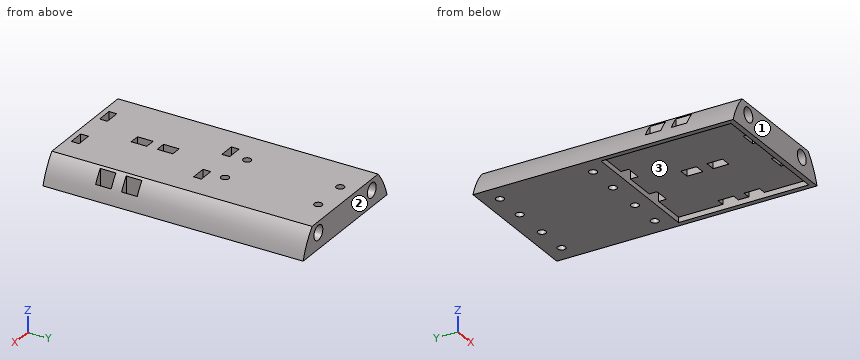
from build123d import *

# Parameters (mm, degrees)
BOSS_EXTRUDE1_DEPTH       = 127
SKETCH10_W                = 62.671930198
SKETCH10_H                = 63.5
CUT_EXTRUDE1_DEPTH        = 2.54
F_1_4_CLEARANCE_HOLE1_D   = 7.14248
F_8_CLEARANCE_HOLE1_D     = 3.8608
SKETCH19_W                = 5.08
SKETCH19_H                = 7.62
SKETCH19_W_2              = 3.81
SKETCH19_W_3              = 7.62
SKETCH19_H_2              = 3.81
CUT_EXTRUDE3_DEPTH        = 14.188436542
F_8_CLEARANCE_HOLE2_D     = 3.8608
F_8_CLEARANCE_HOLE2_DEPTH = 3.81


with BuildPart() as part:
    # Sketch1 → Boss-Extrude1 (new body)
    with BuildSketch(Plane(origin=(0, 0, 0), x_dir=(1, 0, 0), z_dir=(0, 1, 0))):
        with BuildLine():
            Line((-33.875965099, -9.946488053), (33.875965099, -9.946488053))
            ThreePointArc((33.875965099, -9.946488053), (30.982853114, -16.928569016), (26.67, -23.134924595))
            Line((26.67, -23.134924595), (-26.67, -23.134924595))
            ThreePointArc((-26.67, -23.134924595), (-30.982853114, -16.928569016), (-33.875965099, -9.946488053))
        make_face()
    extrude(amount=BOSS_EXTRUDE1_DEPTH)

    # Sketch10 → Cut-Extrude1 (cut)
    with BuildSketch(Plane(origin=(0, 0, 9.946488053), x_dir=(-1, 0, 0), z_dir=(0, 0, -1))):
        with Locations((0, 34.29)):
            Rectangle(SKETCH10_W, SKETCH10_H)
    extrude(amount=-CUT_EXTRUDE1_DEPTH, mode=Mode.SUBTRACT)

    # 1/4 Clearance Hole1 (through all)
    with Locations(Plane(origin=(0, 127, 0), x_dir=(1, 0, 0), z_dir=(0, 1, 0))):
        with Locations((-21.59, -17.810706324), (21.59, -17.810706324)):
            Hole(F_1_4_CLEARANCE_HOLE1_D / 2)

    # #8 Clearance Hole1 (through all)
    with Locations(Plane(origin=(0, 0, 9.946488053), x_dir=(-1, 0, 0), z_dir=(0, 0, -1))):
        with Locations((-8.93698255, 119.253), (-8.93698255, 73.787), (8.93698255, 73.787), (8.93698255, 119.253)):
            Hole(F_8_CLEARANCE_HOLE1_D / 2)

    # Sketch19 → Cut-Extrude3 (cut, through all)
    with BuildSketch(Plane(origin=(0, 0, 9.946488053), x_dir=(-1, 0, 0), z_dir=(0, 0, -1))):
        with Locations((0, 40.64)):
            Rectangle(SKETCH19_W, SKETCH19_H)
        with Locations((0, 27.94)):
            Rectangle(SKETCH19_W, SKETCH19_H)
        with Locations((29.430965099, 40.64)):
            Rectangle(SKETCH19_W_2, SKETCH19_H)
        with Locations((-11.43, 64.135)):
            Rectangle(SKETCH19_W_3, SKETCH19_H_2)
        with Locations((11.43, 64.135)):
            Rectangle(SKETCH19_W_3, SKETCH19_H_2)
        with Locations((-11.43, 4.445)):
            Rectangle(SKETCH19_W_3, SKETCH19_H_2)
        with Locations((11.43, 4.445)):
            Rectangle(SKETCH19_W_3, SKETCH19_H_2)
        with Locations((-29.430965099, 40.64)):
            Rectangle(SKETCH19_W_2, SKETCH19_H)
        with Locations((29.430965099, 27.94)):
            Rectangle(SKETCH19_W_2, SKETCH19_H)
        with Locations((-29.430965099, 27.94)):
            Rectangle(SKETCH19_W_2, SKETCH19_H)
    extrude(amount=-CUT_EXTRUDE3_DEPTH, mode=Mode.SUBTRACT)

    # #8 Clearance Hole2
    with Locations(Plane(origin=(0, 0, 9.946488053), x_dir=(-1, 0, 0), z_dir=(0, 0, -1))):
        with Locations((-24.93898255, 119.253), (-24.93898255, 73.787), (24.93898255, 73.787), (24.93898255, 119.253)):
            Hole(F_8_CLEARANCE_HOLE2_D / 2, depth=F_8_CLEARANCE_HOLE2_DEPTH)


solid = part.part
Geometry: final body of the model. Coordinates: model frame, mm. Face numbers are marked on the shaded views. Give positions to 0.01 mm unless a question says otherwise; leave off trailing zeros. Write each loop counter-clockwise with the first axis right and the second up, starting at its lowest first coordinate (ties: lowest second). Pieces come first, ordered by that corner, then holes. Notation, with made-up numbers: M 68.25,6 L 72.25,6 A24 ccw 72.25,16 Z; hole C -28.75,68 d4. An arc over 180 degrees is marked long. Answer in a Markdown table with one row per item. Add a question column.
(1) First-contact query: pin 1 (6 mm diameter, centred on y = 39.5, z = 20, fed in from +X); pin 2 (2.5 mm diameter, centred on x = 24.94, y = 73.79, fed in from -Z); pin 3 (7 mm diameter, centred on y = 35.5, z = 11.5, fed in from +X). Flat tips, straight axial feed; report the tip coordinate or a pass-through.
(2) Mould query, pull axis Y, two halves, no side actions, for the marked faces 1, 2 and 3. Classes: +Y half, -Y half, draft (parallel to the pull), parting line (faces both ways), or undercut.
(3) Section B-B on y = 41.5. Return loops of the section in (x, z), and give its area (3 significant figures).
(4) Ray query, line 1 (Y direction, x = -0.5, z = 16.75); line 2 (X direction, y = 26.5, z = 17.5); line 3 (Y direction, x = -12, z = 22). Return the intervals inside material, ascending.
(5) Section C-C on x = 0. Return loops of the section in (y, z).
(6) Section D-D on y = 55. Return loops of the section in (x, z).
(7) Section A-A on x = 21.59. Return loops of the section in (y, z), and give its area (3 significant figures).
Result set:
| question | item | result |
|---|---|---|
| 1 | pin 1 | stops at x = 29.99 |
| 1 | pin 2 | stops at z = 13.76 |
| 1 | pin 3 | stops at x = 33.88 |
| 2 | face 1 | -Y half |
| 2 | face 2 | +Y half |
| 2 | face 3 | undercut |
| 3 | outline | M -33.88,9.95 L -31.34,9.95 L -31.34,16.27 A35.31 ccw Z; M -27.53,12.49 L -2.54,12.49 L -2.54,23.13 L -26.67,23.13 A35.31 ccw -27.53,22.11 Z; M 2.54,12.49 L 27.53,12.49 L 27.53,22.11 A35.31 ccw 26.67,23.13 L 2.54,23.13 Z; M 31.34,9.95 L 33.88,9.95 A35.31 ccw 31.34,16.27 Z; hole C -21.59,17.81 d7.14; hole C 21.59,17.81 d7.14 |
| 3 | area | 469 mm^2 |
| 4 | line 1 | y = 0 to 24.13, 31.75 to 36.83, 44.45 to 127 |
| 4 | line 2 | x = -27.53 to -25.15, -18.03 to -2.54, 2.54 to 18.03, 25.15 to 27.53 |
| 4 | line 3 | y = 0 to 2.54, 6.35 to 62.23, 66.04 to 127 |
| 5 | outline | M 0,9.95 L 2.54,9.95 L 2.54,12.49 L 24.13,12.49 L 24.13,23.13 L 0,23.13 Z; M 31.75,12.49 L 36.83,12.49 L 36.83,23.13 L 31.75,23.13 Z; M 44.45,12.49 L 66.04,12.49 L 66.04,9.95 L 127,9.95 L 127,23.13 L 44.45,23.13 Z |
| 6 | outline | M -33.88,9.95 L -31.34,9.95 L -31.34,12.49 L 31.34,12.49 L 31.34,9.95 L 33.88,9.95 A35.31 ccw 26.67,23.13 L -26.67,23.13 A35.31 ccw Z; hole C -21.59,17.81 d7.14; hole C 21.59,17.81 d7.14 |
| 7 | outline | M 0,9.95 L 2.54,9.95 L 2.54,12.49 L 66.04,12.49 L 66.04,9.95 L 127,9.95 L 127,14.24 L 0,14.24 Z; M 0,21.38 L 127,21.38 L 127,23.13 L 0,23.13 Z |
| 7 | area | 607 mm^2 |
